Input: part model. Units: mm. Frame: model coordinates. A direction names the side the tool comes from. Round coordinates to 2 decimals unless told otherwise and drop trailing zeros. Loops run counter-clockwise (first coordinate to the right, second up) from the corner with the lowest first, then second, coordinate; pieces in that order, holes last. Notation, with made-up numbers: (3, -9) -> (52, -9) arc R26 cw to (52, 13) -> close; hole circle Ø3 at (12.25, 45). An arc over 180 degrees is marked (long way). Answer as a JSON object with one key per item and string values.
```python
from build123d import *

# Parameters (mm, degrees)
BOSS_EXTRUDE1_DEPTH = 3.175
FILLET1_R           = 7
FILLET2_R           = 5
SKETCH2_R           = 2.38125
CUT_EXTRUDE1_DEPTH  = 54.908075694
LPATTERN1_COUNT     = 3
LPATTERN1_PITCH     = 12.5


with BuildPart() as part:
    # Sketch1 → Boss-Extrude1 (new body)
    with BuildSketch(Plane.XY):
        with BuildLine():
            Line((-11.618950039, 11), (-36, 11))
            Line((-36, 11), (-36, -29))
            ThreePointArc((-36, -29), (-25, -40), (-14, -29))
            Line((-14, -29), (-14, -11))
            Line((-14, -11), (-11.618950039, -11))
            ThreePointArc((-11.618950039, -11), (16, 0), (-11.618950039, 11))
        make_face()
    extrude(amount=BOSS_EXTRUDE1_DEPTH)

    # Fillet1
    fillet1_edges = [part.edges().sort_by_distance(p)[0] for p in [
        (-36, 11, 1.5875),
    ]]
    fillet(fillet1_edges, radius=FILLET1_R)

    # Fillet2
    # the kernel refuses this fillet: 5 mm, written as the material it adds along each edge
    with BuildSketch(Plane(origin=(-14, -11, 0), x_dir=(1, 0, 0), z_dir=(0, 0, 1))) as fillet2_piece_1:
        with BuildLine():
            CenterArc((5, -4.259237102), FILLET2_R, 121.586822832, 58.413177168)
            Line((0, -4.259237102), (-0.1, -4.259237102))
            Line((-0.1, -4.259237102), (-0.1, 0))
            Line((-0.1, 0), (0, 0.1))
            ThreePointArc((0, 0.1), (1.190524981, 0.1), (2.328670961, 0.085184742))
            Line((2.328670961, 0.085184742), (2.381049961, 0))
        make_face()
    extrude(amount=3.175)

    # Sketch2 → Cut-Extrude1 (cut, through all)
    with BuildSketch(Plane.XY.offset(3.175)):
        Circle(SKETCH2_R)
    cut_extrude1 = extrude(amount=-CUT_EXTRUDE1_DEPTH, mode=Mode.SUBTRACT)

    # LPattern1: Cut-Extrude1 ×3
    with Locations(*[(-i * LPATTERN1_PITCH, 0, 0) for i in range(1, LPATTERN1_COUNT)]):
        add(cut_extrude1, mode=Mode.SUBTRACT)


solid = part.part
```
1) Section C-C, the plane z = 1.75. Output: boundary loops of the cut face in (x, y), plus the area to 3 significant figures.
Output:
{"outline": "(-36, -29) arc R11 ccw to (-14, -29) -> (-14, -15.26) arc R5 cw to (-11.62, -11) arc R16 ccw (long way) to (-11.62, 11) -> (-29, 11) arc R7 ccw to (-36, 4) -> close; hole circle Ø4.76 at (-25, 0); hole circle Ø4.76 at (-12.5, 0); hole circle Ø4.76 at (0, 0)", "area": "1,800 mm^2"}
2) Ray query, probe 1 along Y at (x, z) = (-25, 1.4); probe 2 along Y at (x, z) = (0, 1.25); probe 3 along X at (y, z) = (-28, 1.75). Return the intervals inside material, ascending.
Output:
{"probe 1": "y = -40 to -2.38, 2.38 to 11", "probe 2": "y = -16 to -2.38, 2.38 to 16", "probe 3": "x = -36 to -14"}
3) Section A-A, the plane x = 0. Output: boundary loops of the cut face in (y, z) (3 decimals), plus the area to 3 significant figures.
Output:
{"outline": "(-16, 0) -> (-2.381, 0) -> (-2.381, 3.175) -> (-16, 3.175) -> close; (2.381, 0) -> (16, 0) -> (16, 3.175) -> (2.381, 3.175) -> close", "area": "86.5 mm^2"}
4) Reachability of faces 1 (the face through (-20, 11, 2)), 2 (the face through (-1.89, -1.45, 1.61)), 3 (the face through (-13.35, -12.79, 1.57)) from +Z, -Z, +X, -X, +Y, -Y: full face, straight path, thin tool, end or side. Return the list, or none.
Output:
{"face 1": "+Z, -Z, -X, +Y", "face 2": "+Z, -Z", "face 3": "+Z, -Z, -Y"}
5) Draft query along X for faces 4 (the face through (-14.88, 0.1, 1.61)), 5 (the face through (-15, -5, 0)), 6 (the face through (-33.9, 9, 1.6)). Return one class per face: +X half, -X half, draft (parallel to the pull), parting line (faces both ways), or undercut.
Output:
{"face 4": "undercut", "face 5": "draft", "face 6": "-X half"}
6) Contact query for flat-ended pins moving along their axis: P1, Ø1, axis at x = -15, z = 1.5, coming from the -Y side; P2, Ø4, axis at x = -12.5, y = 0, coming from the +Z side (3 decimals); P3, Ø12, axis at x = -11.5, y = -28, coming from the +Z side (3 decimals). Output: stop coordinate, or through.
Output:
{"P1": "stops at y = -34.55", "P2": "passes through", "P3": "stops at z = 3.175"}
7) Section B-B, the plane y = 0. Output: boundary loops of the cut face in (x, z) (3 decimals), plus the area to 3 significant figures.
Output:
{"outline": "(-36, 0) -> (-27.381, 0) -> (-27.381, 3.175) -> (-36, 3.175) -> close; (-22.619, 0) -> (-14.881, 0) -> (-14.881, 3.175) -> (-22.619, 3.175) -> close; (-10.119, 0) -> (-2.381, 0) -> (-2.381, 3.175) -> (-10.119, 3.175) -> close; (2.381, 0) -> (16, 0) -> (16, 3.175) -> (2.381, 3.175) -> close", "area": "120 mm^2"}
8) Section D-D, the plane y = -12.5. Output: boundary loops of the cut face in (x, z) (1 decimal), plus the area to 3 significant figures.
Output:
{"outline": "(-36, 0) -> (-13.2, 0) -> (-13.2, 3.2) -> (-36, 3.2) -> close; (-10, 0) -> (10, 0) -> (10, 3.2) -> (-10, 3.2) -> close", "area": "136 mm^2"}
